Geometry check sheet. Reference: drawing and pictorial views, mm from the part's lowest x, y, z. A direction names the side the tool comes from. Give positions to 0.01 mm unless a question says otherwise; leave off trailing zeros. Write each loop counter-clockwise with the first axis right and the second up, starting at its lowest first coordinate (ties: lowest second). Pieces come first, ordered by that corner, then holes. Notation, with made-up numbers: (-21, -28.5) -> (-5, -28.5) arc R28 ccw to (-5, -1.5) -> close; hole circle Ø2 at (8, -38). An arc over 180 degrees is marked (long way). Use a Markdown table: item, result. Add a question column.
1. Release check for a two-part mould opening along Y. For the marked faces 1, 2 and 3 record: released by +Y, released by -Y, zero draft, split by the parting line, or undercut.
2. Cross-section at B-B (y = 20.25). Enter the section's corners in (x, z), then the cut area to 3 significant figures.
3. Set-up check for the marked faces 4, 5 and 6: record each of +Z, -Z, +X, -X, +Y, -Y from which the full face is reachable in a straight line by a thin tool's end or side.
4. Cross-section at A-A (x = 6). Enter the section's corners in (y, z).
5. Scan lines: probe 1 along Z at (x, y) = (54, 1.45); probe 2 along X at (y, z) = (14.5, 22); probe 3 along Y at (x, z) = (8, 8.25). Record each from-to range of solid material in increasing order. Write a range as [from, to].
6. Cross-section at C-C (y = 16). Count the separate pieces of the cut face and the enclosed holes in it, then the cut area to 3 significant figures.
7. Gauge pin test, flat ends, axial feed: P1, Ø10, axis at y = 18, z = 12.5, coming from the -X side; P2, Ø7, axis at y = 15, z = 14.5, coming from the -X side; P3, Ø3, axis at y = 10.5, z = 18.5, coming from the +X side; P4, Ø8, axis at x = 27, z = 20.5, coming from the -Y side. Record the tip position at first contact, or that the pin passes through.
8. Cross-section at D-D (z = 27.25). Enter the section's corners in (x, y), then the cut area to 3 significant figures.
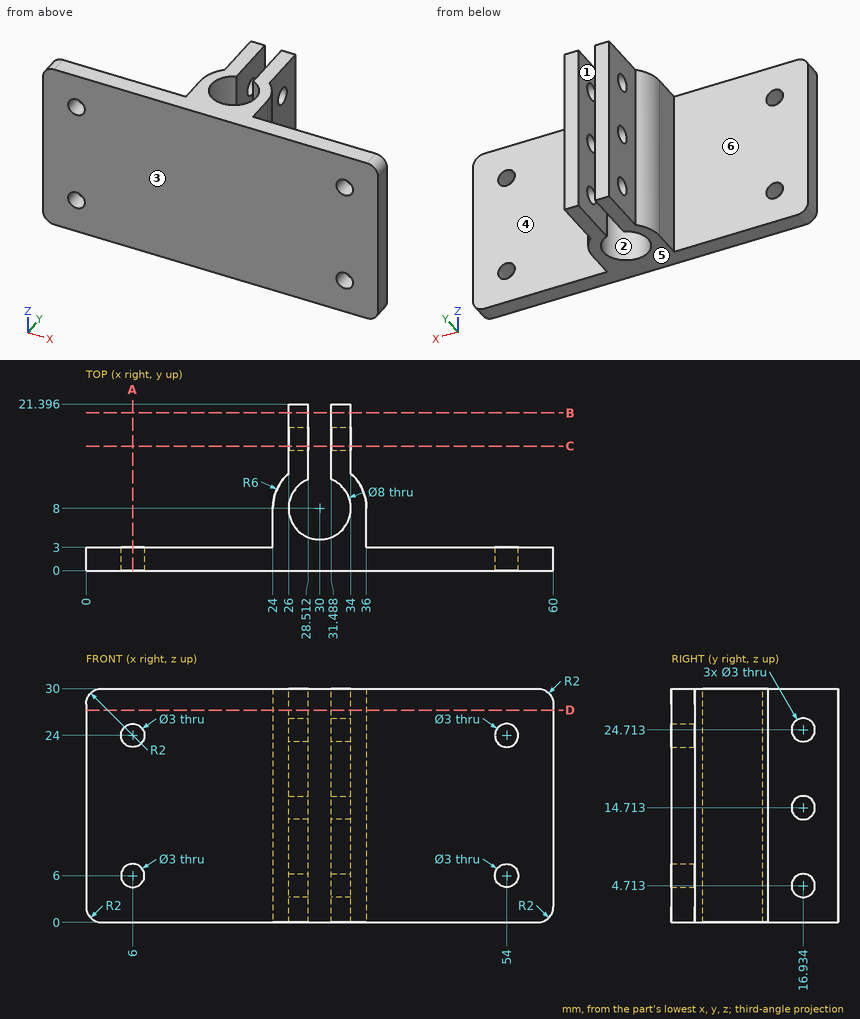
Worked answers:
| question | item | result |
|---|---|---|
| 1 | face 1 | zero draft |
| 1 | face 2 | undercut |
| 1 | face 3 | released by -Y |
| 2 | outline | (26, 0) -> (28.51, 0) -> (28.51, 30) -> (26, 30) -> close; (31.49, 0) -> (34, 0) -> (34, 30) -> (31.49, 30) -> close |
| 2 | area | 151 mm² |
| 3 | face 4 | +Z, -Z, +X, +Y |
| 3 | face 5 | -Z, +X, -X, +Y, -Y |
| 3 | face 6 | +Z, -Z, -X, +Y |
| 4 | outline | (0, 0) -> (3, 0) -> (3, 4.5) -> (0, 4.5) -> close; (0, 7.5) -> (3, 7.5) -> (3, 22.5) -> (0, 22.5) -> close; (0, 25.5) -> (3, 25.5) -> (3, 30) -> (0, 30) -> close |
| 5 | probe 1 | z = [0, 4.5], [7.5, 22.5], [25.5, 30] |
| 5 | probe 2 | x = [26, 28.51], [31.49, 34] |
| 5 | probe 3 | y = [0, 3] |
| 6 | separate pieces | 8 |
| 6 | enclosed holes | 0 |
| 6 | area | 115 mm² |
| 7 | P1 | stops at x = 26 |
| 7 | P2 | stops at x = 25.13 |
| 7 | P3 | stops at x = 35.92 |
| 7 | P4 | stops at y = 0 |
| 8 | outline | (0, 0) -> (60, 0) -> (60, 3) -> (36, 3) -> (36, 8) arc R6 ccw to (34, 12.47) -> (34, 21.4) -> (31.49, 21.4) -> (31.49, 11.71) arc R4 cw (long way) to (28.51, 11.71) -> (28.51, 21.4) -> (26, 21.4) -> (26, 12.47) arc R6 ccw to (24, 8) -> (24, 3) -> (0, 3) -> close |
| 8 | area | 281 mm² |
